```python
from build123d import *

# Parameters (mm, degrees)
F0_W      = 50
F0_H      = 50
F1_DEPTH  = 25
F4_DEPTH  = 70.711678
F5_W      = 50
F5_H      = 50
F6_DEPTH  = 25
F9_SIZE   = 0.5
F11_R     = 2.5
F12_DEPTH = 3


with BuildPart() as f1:
    # F0 (on Top) → F1 (new body)
    with BuildSketch(Plane.XY):
        Rectangle(F0_W, F0_H)
    extrude(amount=F1_DEPTH)

    # F3 (on face) → F4 (cut, through all)
    with BuildSketch(Plane(origin=(25, -25, 0), x_dir=(-0.707107, -0.707107, 0), z_dir=(-0.707107, 0.707107, 0))):
        Polygon((35.355339, 25), (29.015593, 25), (20.355339, 10), (35.355339, 10), align=None)
        Polygon((-20.355339, 10), (-29.015593, 25), (-35.355339, 25), (-35.355339, 10), align=None)
        Polygon((6.122772, 25), (0, 25), (-6.55672, 25), (-15.216974, 10), (14.783026, 10), align=None)
    extrude(amount=F4_DEPTH, mode=Mode.SUBTRACT)

    # F9
    f9_edges = [f1.edges().sort_by_distance(p)[0] for p in [
        (-25, 25, 5),
        (25, 25, 5),
        (25, -25, 5),
        (-25, -25, 5),
        (0, -25, 0),
        (25, 0, 0),
        (0, 25, 0),
        (-25, 0, 0),
    ]]
    chamfer(f9_edges, length=F9_SIZE)

    # F11 (on face) → F12 (cut)
    with BuildSketch(Plane.XY.offset(10)):
        Circle(F11_R)
    extrude(amount=-F12_DEPTH, mode=Mode.SUBTRACT)


with BuildPart() as f6:
    # F5 (on face) → F6 (new body)
    with BuildSketch(Plane.XY.offset(10)):
        Rectangle(F5_W, F5_H)
    extrude(amount=F6_DEPTH)

    # F7: cut F1
    add(f1.part, mode=Mode.SUBTRACT)


with BuildPart() as f6_1:
    # F8: moved
    add(f6.part.moved(Location((55, 0, 0))))


solid = f1.part
```
Model file for the job. Use its own axes, mm. A direction names the side the tool comes from. Coordinates: 2 decimals unless noted, no trailing zeros. Order: outer loops, then holes, each group sorted by start corner. A loop starts at its lowest first (then second) coordinate and runs counter-clockwise, first axis right, second up. Notation, with made-up numbers: (88.25, 72) -> (118.25, 72) arc R25 ccw to (118.25, 106) -> close; hole circle Ø1 at (-25, 27.5). An arc over 180 degrees is marked (long way). Answer as a JSON object with one key per item and string values. Group by question number.
1) Pull direction Z, two halves, no side cores. Call faces 1 (the face through (-0.54, -2.44, 8.52)), 2 (the face through (-18, -18, 10)), 3 (the face through (13, 14, 25)): +Z half, -Z half, draft (parallel to the pull), parting line (faces both ways), or undercut.
2) Cut at B-B, the plane z = 19. Write the cut outline in (x, y), then the cut area to 3 significant figures.
3) Drill centre lines: L1, parallel to Z at x = -21, y = 13.5; L2, parallel to Y at x = 0, z = 8.55; L3, parallel to Z at x = 0, y = 12. Where is each one in solid material? Low to high.
4) Cut at D-D, the plane y = 0. Write the cut outline in (x, z).
5) Flat gauge pins, fed straight in: pin 1 (1.5 mm diameter, centred on x = 0.5, y = 0, fed in from +Z); pin 2 (1 mm diameter, centred on y = -11.5, z = 11.5, fed in from -X); pin 3 (3 mm diameter, centred on x = 12.5, z = 16.5, fed in from +Y). Where does each tip first touch, or does it go through?
6) Cut at C-C, the plane x = 12. Write the cut outline in (y, z), then the cut area to 3 significant figures.
7) Cut at A-A, the plane y = 15. Write the cut outline in (x, z).
8) Which spindle directions (+Z, -Z, +X, -X, +Y, -Y) get a long thin tool onto all of the face, cutting with end or side? Do faces 4 (the face through (0, 0, 7)), 5 (the face through (-7.145, -7.724, 17.395)), 6 (the face through (16.88, 16.583, 15.728)). Say none if no direction does.
Check values:
{
 "1": {"face 1": "draft", "face 2": "undercut", "face 3": "+Z half"},
 "2": {"outline": "(-25, -11.14) -> (-11.14, -25) -> (11.44, -25) -> (-25, 11.44) -> close; (-10.83, 25) -> (25, -10.83) -> (25, 11.14) -> (11.14, 25) -> close", "area": "1,110 mm²"},
 "3": {"L1": "z = 0 to 10", "L2": "y = -25 to -2.5, 2.5 to 25", "L3": "z = 0 to 10, 21.66 to 25"},
 "4": {"outline": "(-25, 0.5) -> (-24.5, 0) -> (24.5, 0) -> (25, 0.5) -> (25, 25) -> (9.27, 25) -> (21.52, 10) -> (2.5, 10) -> (2.5, 7) -> (-2.5, 7) -> (-2.5, 10) -> (-20.91, 10) -> (-8.66, 25) -> (-25, 25) -> close"},
 "5": {"pin 1": "stops at z = 7", "pin 2": "stops at x = -19.16", "pin 3": "stops at y = 23.53"},
 "6": {"outline": "(-25, 0.5) -> (-24.5, 0) -> (24.5, 0) -> (25, 0.5) -> (25, 10) -> (16.79, 10) -> (25, 20.06) -> (25, 25) -> (-2.73, 25) -> (9.52, 10) -> (-25, 10) -> close; (-25, 19.68) -> (-20.66, 25) -> (-25, 25) -> close", "area": "794 mm²"},
 "7": {"outline": "(-25, 0.5) -> (-24.5, 0) -> (24.5, 0) -> (25, 0.5) -> (25, 10) -> (13.79, 10) -> (25, 23.73) -> (25, 25) -> (-5.73, 25) -> (6.52, 10) -> (-25, 10) -> close; (-25, 23.36) -> (-23.66, 25) -> (-25, 25) -> close"},
 "8": {"face 4": "+Z", "face 5": "none", "face 6": "+X, +Y"}
}
